CAD build for the part. Positions are in the model's coordinates, mm. A direction names the side the tool comes from. Coordinates: 2 decimals unless noted, no trailing zeros. Loops run counter-clockwise (first coordinate to the right, second up) from the corner with the lowest first, then second, coordinate; pieces in that order, holes last.
1) Saw through at D-D, the plane x = 14.5. Write the cut outline in (y, z).
2) Two-plate mould, pull along Y, no slides. Class faces 4 (the flat face through (-14, 7, -6)), 5 (the flat face through (-9.614, 6.771, 7.479)), 6 (the cylindrical face through (-12.48, 10.22, 7.48)), 7 (the flat face through (-15.72, 8.27, 7.48)): +Y half, -Y half, draft (parallel to the pull), parting line (faces both ways), or undercut.
3) Saw through at A-A, the plane z = 0. Write the cut outline in (x, y).
4) Wall check: line 1 along Z through (x, y) = (5.5, 7); line 2 along Y through (x, z) = (-30, 10.5); line 3 along X through (y, z) = (8.5, -8). Give the ranges that are in metal, low to high.
5) Which spindle directions (+Z, -Z, +X, -X, +Y, -Y) get a long thin tool onto all of the face, cutting with end or side? Do faces 1 (the cylindrical face through (3.755, 1.521, 11.923)), 2 (the flat face through (-3, 27, 13)), 3 (the flat face through (-9.614, 6.771, -7.521)). Say none if no direction does.
6) Pin check, flat tips, straight feed: pin 1 Ø3 at (x, z) = (1.5, -19.5) entering from +Y; pin 2 Ø5 at (x, y) = (11, 9) entering from -Z; pin 3 Ø5 at (x, z) = (19.5, -12) entering from +Y. Stop position of each tip, or through.
7) Saw through at B-B, the plane x = 0. Write the cut outline in (y, z), and give its area (3 significant figures).
8) Saw through at C-C, the plane y = 34.5. Write the cut outline in (x, z), and give its area (3 significant figures).
```python
from build123d import *

# Parameters (mm, degrees)
SKETCH_1_R          = 34.5
EXTRUDE_1_DEPTH     = 3
SKETCH_2_R          = 12.5
CUT_EXTRUDE_1_DEPTH = 3
EXTRUDE_START       = 6
SKETCH_3_R          = 1.183017338
EXTRUDE_2_DEPTH     = 3
EXTRUDE_START_2     = -9
SKETCH_3_2_R        = 1.183017338
EXTRUDE_3_DEPTH     = 3
EXTRUDE_START_3     = 10
SKETCH_4_W          = 40.46646749
SKETCH_4_H          = 46.577480255
EXTRUDE_6_DEPTH     = 3
SKETCH_5_R          = 7.75
CUT_EXTRUDE_2_DEPTH = 3
SKETCH_6_W          = 23.274927202
SKETCH_6_H          = 9.540013766
EXTRUDE_7_DEPTH     = 17


with BuildPart() as part:
    # Sketch 1 → Extrude 1 (new body)
    with BuildSketch(Plane(origin=(0, 0, 0), x_dir=(1, 0, 0), z_dir=(0, 1, 0))):
        with Locations(Location((0, 0, 0), (0, 0, 270))):
            Circle(SKETCH_1_R)
    extrude(amount=EXTRUDE_1_DEPTH)

    # Sketch 2 → Cut-Extrude 1 (cut)
    with BuildSketch(Plane(origin=(0, 3, 0), x_dir=(1, 0, 0), z_dir=(0, 1, 0))):
        with Locations(Location((0, 0, 0), (0, 0, 270))):
            Circle(SKETCH_2_R)
    extrude(amount=-CUT_EXTRUDE_1_DEPTH, mode=Mode.SUBTRACT)

    # Sketch 3 → Extrude 2 (add)
    with BuildSketch(Plane.XY.offset(EXTRUDE_START)):
        Polygon((-12.5, 3), (-6.645761315, 10.649339614), (-10.240290901, 13.400326656), (-21.352795206, 3), align=None)
        with Locations((-11.606709205, 9.420794795)):
            Circle(SKETCH_3_R, mode=Mode.SUBTRACT)
    extrude_2 = extrude(amount=EXTRUDE_2_DEPTH)

    # Sketch 3_2 → Extrude 3 (add)
    with BuildSketch(Plane.XY.offset(EXTRUDE_START_2)):
        Polygon((-12.5, 3), (-6.645761315, 10.649339614), (-10.240290901, 13.400326656), (-21.352795206, 3), align=None)
        with Locations((-11.606709205, 9.420794795)):
            Circle(SKETCH_3_2_R, mode=Mode.SUBTRACT)
    extrude_3 = extrude(amount=EXTRUDE_3_DEPTH)

    # Mirror 1: Extrude 2, Extrude 3 across plane
    add(extrude_2.mirror(Plane(origin=(0, 0, 0), x_dir=(0, 0, 1), z_dir=(1, 0, 0))))
    add(extrude_3.mirror(Plane(origin=(0, 0, 0), x_dir=(0, 0, 1), z_dir=(1, 0, 0))))

    # Sketch 4 → Extrude 6 (add)
    with BuildSketch(Plane.XY.offset(EXTRUDE_START_3)):
        with Locations((-2.561924873, 26.288740128)):
            Rectangle(SKETCH_4_W, SKETCH_4_H)
    extrude(amount=EXTRUDE_6_DEPTH)

    # Sketch 5 → Cut-Extrude 2 (cut)
    with BuildSketch(Plane.XY.offset(13)):
        with Locations((-2.710861026, 36.508686197)):
            Circle(SKETCH_5_R)
    extrude(amount=-CUT_EXTRUDE_2_DEPTH, mode=Mode.SUBTRACT)

    # Sketch 6 → Extrude 7 (add)
    with BuildSketch(Plane(origin=(0, 3, 0), x_dir=(1, 0, 0), z_dir=(0, 1, 0))):
        with Locations((0, 21.989393432)):
            Rectangle(SKETCH_6_W, SKETCH_6_H)
    extrude(amount=EXTRUDE_7_DEPTH)


solid = part.part
```
Data:
1. outline: (0, -31.3) - (3, -31.3) - (3, -9) - (9.41, -9) - (9.41, -6) - (3, -6) - (3, 6) - (9.41, 6) - (9.41, 9) - (3, 9) - (3, 10) - (49.58, 10) - (49.58, 13) - (3, 13) - (3, 31.3) - (0, 31.3) - close
2. face 4: draft
2. face 5: undercut
2. face 6: undercut
2. face 7: +Y half
3. outline: (-34.5, 0) - (-12.5, 0) - (-12.5, 3) - (-34.5, 3) - close; (12.5, 0) - (34.5, 0) - (34.5, 3) - (12.5, 3) - close
4. line 1: z = -26.76 to -17.22, 10 to 13
4. line 2: y = 0 to 3
4. line 3: x = -15.48 to -12.35, -10.86 to -8.29, 8.29 to 10.86, 12.35 to 15.48
5. face 1: -Y
5. face 2: +Z, +X, -X, +Y
5. face 3: none
6. pin 1: stops at y = 20
6. pin 2: stops at z = -26.76
6. pin 3: stops at y = 3
7. outline: (0, -34.5) - (3, -34.5) - (3, -26.76) - (20, -26.76) - (20, -17.22) - (3, -17.22) - (3, -12.5) - (0, -12.5) - close; (0, 12.5) - (3, 12.5) - (3, 10) - (29.25, 10) - (29.25, 13) - (3, 13) - (3, 34.5) - (0, 34.5) - close; (43.77, 10) - (49.58, 10) - (49.58, 13) - (43.77, 13) - close
7. area: 390 mm2
8. outline: (-22.8, 10) - (-10.2, 10) - (-10.2, 13) - (-22.8, 13) - close; (4.77, 10) - (17.67, 10) - (17.67, 13) - (4.77, 13) - close
8. area: 76.5 mm2
